from build123d import *

# Parameters (mm, degrees)
F0_W     = 38.1
F0_H     = 19.05
F0_H_2   = 19.0520574
F1_DEPTH = 152.4


# Not quite as in the source:
# - ends of sketch curves that miss each other by under 0.0002 mm in the source are joined


with BuildPart() as f1:
    # F0 (on Front) → F1 (new body)
    with BuildSketch(Plane.XZ):
        with Locations((14.288262, -9.5260414)):
            Rectangle(F0_W, F0_H)
        with BuildLine():
            Line((-14.287246, -19.0510414), (-4.761738, -19.0510414))
            Line((-4.761738, -19.0510414), (-4.761738, -0.0010414))
            Line((-4.761738, -0.0010414), (-4.761738, 19.051016))
            Line((-4.761738, 19.051016), (-23.812754, 19.051016))
            ThreePointArc((-23.812754, 19.051016), (-30.548305301, 16.261059301), (-33.338262, 9.525508))
            ThreePointArc((-33.338262, 9.525508), (-30.548305301, 2.789956699), (-23.812754, 0))
            Line((-23.812754, 0), (-23.812754, -6.3503556))
            Line((-23.812754, -6.3503556), (-20.6375762, -6.3503556))
            ThreePointArc((-20.6375762, -6.3503556), (-19.9375622279, -9.969300362), (-17.4624299923, -12.700695633))
            ThreePointArc((-17.4624299923, -12.700695633), (-14.947472994, -15.4121856415), (-14.287246, -19.0510414))
        make_face()
        with Locations((14.288262, 9.5249873)):
            Rectangle(F0_W, F0_H_2)
    extrude(amount=F1_DEPTH)


solid = f1.part
Work out the finished part from the listing and answer in its coordinate system (mm). A direction names the side the tool comes from. Give positions to 0.01 mm unless a question says otherwise; leave off trailing zeros. Order: outer loops, then holes, each group sorted by start corner. A loop starts at its lowest first (then second) coordinate and runs counter-clockwise, first axis right, second up. Notation, with made-up numbers: (19.25, -6.75) - (55.25, -6.75) arc R16 cw to (55.25, 9.25) - close; hole circle Ø4 at (-36, 73). An arc over 180 degrees is marked (long way). Answer as CSV lines item,"result". Start each with the question number.
Q1. The part is cut by section B-B (z = -9.5). Write down the section's boundary in (x, y), then the cut area to 3 significant figures.
Q2. Find the intervals of material crossed by L1, parallel to Z at x = -24.5, y = -58; L2, parallel to X at y = -26, z = -4; L3, parallel to X at y = -62, z = 4, in increasing order. Write a range as [from, to].
Q3. The part is cut by section A-A (y = -32.5). Write down the section's boundary in (x, z), then the cut area to 3 significant figures.
Q4. For faces 1 (the face through (0, 0, 0)), 2 (the face through (-23.813, -75, -3)), determine the directions among +Z, -Z, +X, -X, +Y, -Y from which every point of the face is accessible in a straight line to the end or side of a thin tool.
Q5. Given pin 1 Ø1.5 at (y, z) = (-33.5, 4.5) entering from -X; pin 2 Ø1.6 at (x, y) = (-22.5, -45.5) entering from -Z; pin 3 Ø2 at (y, z) = (-53.5, 6.5) entering from -X, each flat-ended and moving along its own axis, determine where each tip first touches the part or whether it passes through.
Check result:
1,outline,"(-20.15, -152.4) - (33.34, -152.4) - (33.34, 0) - (-20.15, 0) - close"
1,area,"8,150 mm²"
2,L1,"z = [0.02, 19.03]"
2,L2,"x = [-23.81, 33.34]"
2,L3,"x = [-31.57, 33.34]"
3,outline,"(-23.81, -6.35) - (-20.64, -6.35) arc R6.85 ccw to (-17.46, -12.7) arc R6.6 cw to (-14.29, -19.05) - (33.34, -19.05) - (33.34, 19.05) - (-23.81, 19.05) arc R9.53 ccw to (-23.81, 0) - close"
3,area,"2,240 mm²"
4,face 1,"+Z, -Z, +X, -X, +Y"
4,face 2,"-Z, -X, +Y, -Y"
5,pin 1,"stops at x = -32.32"
5,pin 2,"stops at z = -6.35"
5,pin 3,"stops at x = -33.12"
